Source: CAD feature listing. Evaluate the final solid. Frame: model axes, mm. Face numbers are marked on the shaded views. Give positions to 0.01 mm unless a question says otherwise; leave off trailing zeros. Loops run counter-clockwise (first coordinate to the right, second up) from the corner with the lowest first, then second, coordinate; pieces in that order, holes last. Notation, with made-up numbers: M -10,60.25 L 29,60.25 A33 cw 29,93.25 Z; hole C 1,13.25 d11. An arc over 180 degrees is marked long. Answer in a Markdown table with one row per item.
```python
from build123d import *

# Parameters (mm, degrees)
SKETCH_1_W          = 430
SKETCH_1_H          = 70
EXTRUDE_1_DEPTH     = 8
FILLET_1_R          = 1
SKETCH_2_W          = 390
SKETCH_2_H          = 2.5
EXTRUDE_2_DEPTH     = 10
SKETCH_3_R          = 1.65
SKETCH_3_R_2        = 3.25
SKETCH_3_R_3        = 5.7
SKETCH_3_R_4        = 4.7
SKETCH_3_R_5        = 1.7
SKETCH_3_R_6        = 2
SKETCH_3_R_7        = 3.2
CUT_EXTRUDE_1_DEPTH = 19
CUT_EXTRUDE_2_DEPTH = 4.5
SKETCH_5_R          = 3.5
CUT_EXTRUDE_3_DEPTH = 2
SKETCH_6_R          = 8.25
CUT_EXTRUDE_4_DEPTH = 19
SKETCH_7_R          = 20
CUT_EXTRUDE_5_DEPTH = 4


with BuildPart() as part:
    # 草圖1 → 填料-伸長1 (new body)
    with BuildSketch(Plane.XY):
        Rectangle(SKETCH_1_W, SKETCH_1_H)
    extrude(amount=EXTRUDE_1_DEPTH)

    # 圓角1
    fillet_1_edges = [part.edges().sort_by_distance(p)[0] for p in [
        (215, -35, 4),
        (-215, -35, 4),
        (-215, 35, 4),
        (215, 35, 4),
    ]]
    fillet(fillet_1_edges, radius=FILLET_1_R)

    # 草圖2 → 填料-伸長2 (add)
    with BuildSketch(Plane.XY.offset(8)):
        with Locations((0, 29.75)):
            Rectangle(SKETCH_2_W, SKETCH_2_H)
        with Locations((0, -29.75)):
            Rectangle(SKETCH_2_W, SKETCH_2_H)
    extrude(amount=EXTRUDE_2_DEPTH)

    # 草圖3 → 除料-伸長1 (cut, through all)
    with BuildSketch(Plane(origin=(0, 0, 0), x_dir=(-1, 0, 0), z_dir=(0, 0, -1))):
        with Locations((90.1, 2.4)):
            Circle(SKETCH_3_R)
        with BuildLine():
            ThreePointArc((111, -7.5), (110.23508972, -3.469747103), (108.04673847, 0))
            Line((108.04673847, 0), (91.95326153, 0))
            ThreePointArc((91.95326153, 0), (95.969747103, -17.73508972), (111, -7.5))
        make_face()
        with BuildLine():
            Line((91.95326153, 0), (108.04673847, 0))
            ThreePointArc((108.04673847, 0), (100, 3.5), (91.95326153, 0))
        make_face()
        with Locations((109.9, -17.4)):
            Circle(SKETCH_3_R)
        with Locations((80, -16.75)):
            Circle(SKETCH_3_R_2)
        with Locations((45, -10.11)):
            Circle(SKETCH_3_R_3)
        with Locations((160, 0)):
            Circle(SKETCH_3_R_4)
        with Locations((160, -9)):
            Circle(SKETCH_3_R_5)
        with BuildLine():
            ThreePointArc((155.3, 0), (160, -4.7), (164.7, 0))
            Line((164.7, 0), (155.3, 0))
        make_face()
        with BuildLine():
            Line((155.3, 0), (164.7, 0))
            ThreePointArc((164.7, 0), (160, 4.7), (155.3, 0))
        make_face()
        with Locations((65, -17.2)):
            Circle(SKETCH_3_R_6)
        with Locations((65, -7.2)):
            Circle(SKETCH_3_R_7)
    extrude(amount=-CUT_EXTRUDE_1_DEPTH, mode=Mode.SUBTRACT)

    # 草圖4 → 除料-伸長2 (cut)
    with BuildSketch(Plane(origin=(0, 0, 0), x_dir=(-1, 0, 0), z_dir=(0, 0, -1))):
        with BuildLine():
            Line((45, 7.5), (105, 7.5))
            ThreePointArc((105, 7.5), (120, -7.5), (105, -22.5))
            Line((105, -22.5), (45, -22.5))
            ThreePointArc((45, -22.5), (30, -7.5), (45, 7.5))
        make_face()
    extrude(amount=-CUT_EXTRUDE_2_DEPTH, mode=Mode.SUBTRACT)

    # 草圖5 → 除料-伸長3 (cut)
    with BuildSketch(Plane(origin=(0, 0, 4.5), x_dir=(-1, 0, 0), z_dir=(0, 0, -1))):
        with Locations((65, -17.2)):
            Circle(SKETCH_5_R)
    extrude(amount=-CUT_EXTRUDE_3_DEPTH, mode=Mode.SUBTRACT)

    # 草圖6 → 除料-伸長4 (cut, through all)
    with BuildSketch(Plane(origin=(0, 0, 0), x_dir=(-1, 0, 0), z_dir=(0, 0, -1))):
        with Locations((-165, 0)):
            Circle(SKETCH_6_R)
    extrude(amount=-CUT_EXTRUDE_4_DEPTH, mode=Mode.SUBTRACT)

    # 草圖7 → 除料-伸長5 (cut)
    with BuildSketch(Plane(origin=(0, 0, 0), x_dir=(-1, 0, 0), z_dir=(0, 0, -1))):
        with Locations((160, 0.609446204)):
            Circle(SKETCH_7_R)
    extrude(amount=-CUT_EXTRUDE_5_DEPTH, mode=Mode.SUBTRACT)


solid = part.part
```
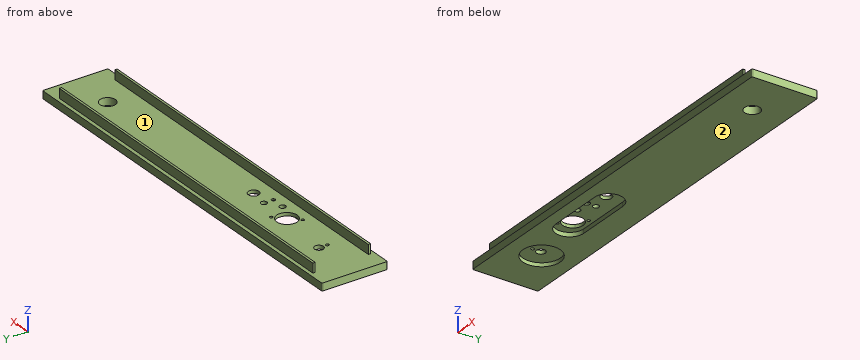
1) Section C-C, the plane x = 90. Return loops of the section in (y, z), then the cut area to 3 significant figures.
Reply:
| item | result |
|---|---|
| outline | M -35,0 L 35,0 L 35,8 L 31,8 L 31,18 L 28.5,18 L 28.5,8 L -28.5,8 L -28.5,18 L -31,18 L -31,8 L -35,8 Z |
| area | 610 mm² |
2) Section B-B, the plane z = 11.25. Return loops of the section in (x, y).
Reply:
| item | result |
|---|---|
| outline | M -195,-31 L 195,-31 L 195,-28.5 L -195,-28.5 Z; M -195,28.5 L 195,28.5 L 195,31 L -195,31 Z |
3) Section D-D, the plane x = -95.5. Return loops of the section in (y, z).
Reply:
| item | result |
|---|---|
| outline | M -35,0 L -22.5,0 L -22.5,4.5 L -17.54,4.5 L -17.54,8 L -28.5,8 L -28.5,18 L -31,18 L -31,8 L -35,8 Z; M 2.54,4.5 L 7.5,4.5 L 7.5,0 L 35,0 L 35,8 L 31,8 L 31,18 L 28.5,18 L 28.5,8 L 2.54,8 Z |
4) Pin query (flat end, axial travel): pin 1 Ø3 at (y, z) = (-29.5, 11) entering from -X; pin 2 Ø1 at (x, z) = (-2.5, 16) entering from -Y; pin 3 Ø2 at (x, y) = (3, -21.5) entering from +Z; pin 4 Ø5 at (y, z) = (-2, 9) entering from -X. Return the tip coordinate at first contact, or that it passes through.
Reply:
| item | result |
|---|---|
| pin 1 | stops at x = -195 |
| pin 2 | stops at y = -31 |
| pin 3 | stops at z = 8 |
| pin 4 | stops at x = -215 |
5) Material intervals for L1, parallel to Y at x = -65, z = 5.55; L2, parallel to X at y = -10.5, z = 6.5; L3, parallel to Y at x = 112, z = 14.25, sorted ascending.
Reply:
| item | result |
|---|---|
| L1 | y = -35 to -20.7, -13.7 to -10.4, -4 to 35 |
| L2 | x = -215 to -160.8, -159.2 to -110.58, -89.42 to -50.69, -39.31 to 215 |
| L3 | y = -31 to -28.5, 28.5 to 31 |
6) Pull-direction query (Y, two-part tool) for the marked faces 1 and 2; classes: released by +Y, released by -Y, zero draft, split by the parting line, or undercut.
Reply:
| item | result |
|---|---|
| face 1 | undercut |
| face 2 | zero draft |
7) Section A-A, the plane x = 165. Return loops of the section in (y, z).
Reply:
| item | result |
|---|---|
| outline | M -35,0 L -8.25,0 L -8.25,8 L -28.5,8 L -28.5,18 L -31,18 L -31,8 L -35,8 Z; M 8.25,0 L 35,0 L 35,8 L 31,8 L 31,18 L 28.5,18 L 28.5,8 L 8.25,8 Z |
